Work out the finished part from the listing and answer in its coordinate system (mm). A direction names the side the tool comes from. Coordinates: 2 decimals unless noted, no trailing zeros. Order: outer loops, then holes, each group sorted by start corner. A loop starts at its lowest first (then second) coordinate and runs counter-clockwise, first axis right, second up. Notation, with made-up numbers: M 70,59 L 121,59 A19 ccw 121,79 Z; hole C 83,52 d5. An arc over 180 degrees is marked long. Answer in a Markdown table with one row per item. Add a question column.
Item 1: The mould has two halves that part along Z. Classify faces 1 (the face through (0, -17.423, -1)), 2 (the face through (7, -28, -7)), 3 (the face through (-2.26, 17.806, -18.241)), 4 (the face through (-7.594, 12.115, -18.241)): released by +Z, released by -Z, zero draft, split by the parting line, or undercut.
Item 2: The part is cut by section B-B (x = 18). Write down the section's boundary in (y, z), then the cut area to 3 significant figures.
Item 3: Consider line 1 (Y direction, x = -2.5, z = -1.5); line 2 (Y direction, x = 0, z = -33); line 3 (Z direction, x = -8, y = 22). Determine where each line is inside the solid, lowest interval first. Write a range as from..to.
Item 4: The part is cut by section D-D (x = -24). Write down the section's boundary in (y, z).
Item 5: Which of the six approach directions +Z, -Z, +X, -X, +Y, -Y give full straight-line access (tool end or side, diameter ignored) to faces 5 (the face through (12, -6.423, 1)), 6 (the face through (-8.5, -29, -3)), 7 (the face through (0, -20, -2.5)), 8 (the face through (-7, -28, -7))?
Item 6: The part is cut by section A-A (y = -13.5). Write down the section's boundary in (x, z), then the cut area to 3 significant figures.
Item 7: The part is cut by section C-C (y = 19). Write down the section's boundary in (x, z).
Item 8: Flat-ended cylindrical pins translate along their axes: pin 1 Ø8 at (x, z) = (-16.5, -3) entering from +Y; pin 2 Ø4.5 at (y, z) = (18.5, -21) entering from -X; pin 3 Ø2.5 at (y, z) = (-32, -0.5) entering from +X; pin 4 Ø2 at (y, z) = (-28.5, 1.5) entering from -X. Find the tip coordinate at first contact, or state that the pin passes through.
from build123d import *

# Parameters (mm, degrees)
BOSS_EXTRUDE1_DEPTH             = 2
SKETCH2_R                       = 0.75
BOSS_EXTRUDE2_DEPTH             = 1.5
BOSS_EXTRUDE3_REACH             = 75.225
BOSS_EXTRUDE3_DIRECTION_2_REACH = 75.225
CUT_EXTRUDE1_DEPTH              = 16.5
SKETCH5_W                       = 2.5
SKETCH5_H                       = 22
BOSS_EXTRUDE4_DEPTH             = 7
SKETCH6_W                       = 12
SKETCH6_H                       = 3
SKETCH6_W_2                     = 22
SKETCH6_H_2                     = 4.5
CUT_EXTRUDE2_DEPTH              = 2.5
SKETCH7_W                       = 12
SKETCH7_H                       = 7
SKETCH7_H_2                     = 4.5
BOSS_EXTRUDE5_DEPTH             = 2.5
FILLET1_R                       = 4
FILLET2_R                       = 1


with BuildPart() as part:
    # Sketch1 → Boss-Extrude1 (new body)
    with BuildSketch(Plane.XY):
        with BuildLine():
            Line((-28.565713714, 28), (28.565713714, 28))
            ThreePointArc((28.565713714, 28), (39.988956848, 0.93985647), (29.849608312, -26.627070504))
            Line((29.849608312, -26.627070504), (9, -50))
            Line((9, -50), (-9, -50))
            Line((-9, -50), (-29.849608312, -26.627070504))
            ThreePointArc((-29.849608312, -26.627070504), (-39.988956848, 0.93985647), (-28.565713714, 28))
        make_face()
        with BuildLine():
            Line((7, -6.422616289), (15, -6.422616289))
            Line((15, -6.422616289), (15, -17.422616289))
            Line((15, -17.422616289), (-15, -17.422616289))
            Line((-15, -17.422616289), (-15, -6.422616289))
            Line((-15, -6.422616289), (-7, -6.422616289))
            ThreePointArc((-7, -6.422616289), (0, 9.5), (7, -6.422616289))
        make_face(mode=Mode.SUBTRACT)
    extrude(amount=BOSS_EXTRUDE1_DEPTH)

    # Sketch2 → Boss-Extrude2 (add, symmetric)
    with BuildSketch(Plane(origin=(0, 0, 0), x_dir=(0, 0, -1), z_dir=(1, 0, 0))):
        Polygon((0, 9.5), (37, 20), (37, 28), (0, 28), align=None)
        with Locations((3, 26)):
            Circle(SKETCH2_R, mode=Mode.SUBTRACT)
        with Locations((6, 26)):
            Circle(SKETCH2_R, mode=Mode.SUBTRACT)
        with Locations((9, 26)):
            Circle(SKETCH2_R, mode=Mode.SUBTRACT)
        with Locations((12, 26)):
            Circle(SKETCH2_R, mode=Mode.SUBTRACT)
        with Locations((15, 26)):
            Circle(SKETCH2_R, mode=Mode.SUBTRACT)
        with Locations((18, 26)):
            Circle(SKETCH2_R, mode=Mode.SUBTRACT)
        with Locations((21, 26)):
            Circle(SKETCH2_R, mode=Mode.SUBTRACT)
        with Locations((24, 26)):
            Circle(SKETCH2_R, mode=Mode.SUBTRACT)
        with Locations((27, 26)):
            Circle(SKETCH2_R, mode=Mode.SUBTRACT)
        with Locations((30, 26)):
            Circle(SKETCH2_R, mode=Mode.SUBTRACT)
        with Locations((33, 26)):
            Circle(SKETCH2_R, mode=Mode.SUBTRACT)
    extrude(amount=BOSS_EXTRUDE2_DEPTH, both=True)

    # Boss-Extrude3: up to this plane
    boss_extrude3_end = Plane(origin=(1.5, 20, -37), z_dir=(0, 0, 1))
    # Sketch3 → Boss-Extrude3 (add, up to the surface)
    with BuildSketch(Plane(origin=(0, 0.708044617, -2.495014365), x_dir=(1, 0, 0), z_dir=(0, -0.27300368557463345, 0.9620129872629926)), mode=Mode.PRIVATE) as boss_extrude3_sk1:
        Polygon((1, 9.088350078), (-1, 9.088350078), (-9.380481154, -0.899118445), (-12.061636705, 1.350638189), (-3, 12.149876287), (3, 12.149876287), (12.061636705, 1.350638189), (9.380481154, -0.899118445), align=None)
    boss_extrude3_tool1 = split(extrude(boss_extrude3_sk1.sketch, amount=-BOSS_EXTRUDE3_REACH, mode=Mode.PRIVATE), bisect_by=boss_extrude3_end, keep=Keep.BOTH, mode=Mode.PRIVATE)
    add(boss_extrude3_tool1.solids().sort_by_distance((0, 9.715001, 0.061014))[0])

    # Boss-Extrude3 direction 2: up to this plane
    boss_extrude3_direction_2_end = Plane(origin=(0, 0, 2), z_dir=(0, 0, 1))
    # Sketch3 → Boss-Extrude3 direction 2 (add, up to the surface)
    with BuildSketch(Plane(origin=(0, 0.708044617, -2.495014365), x_dir=(1, 0, 0), z_dir=(0, -0.27300368557463345, 0.9620129872629926)), mode=Mode.PRIVATE) as boss_extrude3_direction_2_sk1:
        Polygon((1, 9.088350078), (-1, 9.088350078), (-9.380481154, -0.899118445), (-12.061636705, 1.350638189), (-3, 12.149876287), (3, 12.149876287), (12.061636705, 1.350638189), (9.380481154, -0.899118445), align=None)
    boss_extrude3_direction_2_tool1 = split(extrude(boss_extrude3_direction_2_sk1.sketch, amount=BOSS_EXTRUDE3_DIRECTION_2_REACH, mode=Mode.PRIVATE), bisect_by=boss_extrude3_direction_2_end, keep=Keep.BOTH, mode=Mode.PRIVATE)
    add(boss_extrude3_direction_2_tool1.solids().sort_by_distance((0, 9.715001, 0.061014))[0])

    # Sketch4 → Cut-Extrude1 (cut, symmetric)
    with BuildSketch(Plane(origin=(0, 0, 0), x_dir=(0, 0, -1), z_dir=(1, 0, 0))):
        Polygon((20.376494071, 1.70865423), (25.234329822, 8.565064446), (31.144411196, 4.377712218), align=None)
    extrude(amount=CUT_EXTRUDE1_DEPTH, both=True, mode=Mode.SUBTRACT)

    # Sketch5 → Boss-Extrude4 (add)
    with BuildSketch(Plane(origin=(0, 0, 0), x_dir=(-1, 0, 0), z_dir=(0, 0, -1))):
        with Locations((-7.25, -28.422616289)):
            Rectangle(SKETCH5_W, SKETCH5_H)
        with Locations((7.25, -28.422616289)):
            Rectangle(SKETCH5_W, SKETCH5_H)
    extrude(amount=BOSS_EXTRUDE4_DEPTH)

    # Sketch6 → Cut-Extrude2 (cut)
    with BuildSketch(Plane.XY.offset(2)):
        with Locations((0, -23.422616289)):
            Rectangle(SKETCH6_W, SKETCH6_H)
        with Locations((0, -28.672616289)):
            Rectangle(SKETCH6_W_2, SKETCH6_H_2)
    extrude(amount=-CUT_EXTRUDE2_DEPTH, mode=Mode.SUBTRACT)

    # Sketch7 → Boss-Extrude5 (add)
    with BuildSketch(Plane(origin=(0, 0, 0), x_dir=(-1, 0, 0), z_dir=(0, 0, -1))):
        with Locations((0, -28.422616289)):
            Rectangle(SKETCH7_W, SKETCH7_H)
        with Locations((0, -19.672616289)):
            Rectangle(SKETCH7_W, SKETCH7_H_2)
    extrude(amount=BOSS_EXTRUDE5_DEPTH)

    # Fillet1
    # the kernel refuses this fillet: 4 mm, written as the material it adds along each edge
    with BuildSketch(Plane(origin=(-6, -31.922616289, 0), x_dir=(0, 0, -1), z_dir=(1, 0, 0))) as fillet1_piece_1:
        with BuildLine():
            CenterArc((4, -3.708099244), FILLET1_R, 112.024312837, 67.975687163)
            Line((0, -3.708099244), (-0.08, -3.708099244))
            Line((-0.08, -3.708099244), (-0.08, 0))
            Line((-0.08, 0), (0, 0.08))
            ThreePointArc((0, 0.08), (1.25, 0.08), (2.47, 0.074161985))
            Line((2.47, 0.074161985), (2.5, 0))
        make_face()
    extrude(amount=12)

    # Fillet2
    fillet2_edges = [part.edges().sort_by_distance(p)[0] for p in [
        (7, -6.422616289, 1),
        (-7, -6.422616289, 1),
    ]]
    fillet(fillet2_edges, radius=FILLET2_R)


solid = part.part
Reply:
| question | item | result |
|---|---|---|
| 1 | face 1 | zero draft |
| 1 | face 2 | released by -Z |
| 1 | face 3 | undercut |
| 1 | face 4 | undercut |
| 2 | outline | M -39.91,0 L 28,0 L 28,2 L -39.91,2 Z |
| 2 | area | 136 mm2 |
| 3 | line 1 | y = -32.51..-24.92, -21.92..-17.42, 8.01..13.06 |
| 3 | line 2 | y = 18.81..25.25, 26.75..28 |
| 3 | line 3 | z = 0..2 |
| 4 | outline | M -33.18,0 L 28,0 L 28,2 L -33.18,2 Z |
| 5 | face 5 | +Z, -Z |
| 5 | face 6 | -Z, -X, -Y |
| 5 | face 7 | -Z, -Y |
| 5 | face 8 | -Z, +X, -X, -Y |
| 6 | outline | M -37.65,0 L -15,0 L -15,2 L -37.65,2 Z; M 15,0 L 37.65,0 L 37.65,2 L 15,2 Z |
| 6 | area | 90.6 mm2 |
| 7 | outline | M -35.2,0 L -1.5,0 L -1.5,-22.45 L -3,-22.45 L -6.33,-37 L -1.76,-37 L -1,-33.66 L 1,-33.66 L 1.76,-37 L 6.33,-37 L 3,-22.45 L 1.5,-22.45 L 1.5,0 L 35.2,0 L 35.2,2 L -35.2,2 Z |
| 8 | pin 1 | stops at y = 28 |
| 8 | pin 2 | stops at x = -4.96 |
| 8 | pin 3 | stops at x = 26.08 |
| 8 | pin 4 | stops at x = -29.07 |
